Geometry check sheet. Reference: the model listing, model coordinates, mm. Face numbers are marked on the shaded views. Give positions to 0.01 mm unless a question says otherwise; leave off trailing zeros. Order: outer loops, then holes, each group sorted by start corner. A loop starts at its lowest first (then second) coordinate and runs counter-clockwise, first axis right, second up. Notation, with made-up numbers: M -17,-4.75 L -6,-4.75 A17 ccw -6,16.25 Z; hole C -21.5,29.5 d1. An arc over 180 degrees is marked long. Answer as CSV lines item,"result". Start each with the question number.
Q1. Section check A-A, the plane x = 0. Record the boundary of the cut face in (y, z).
Q2. Mould release check, pull along X, two halves, no side actions. Record for the marked faces 1 and 2: +X half, -X half, draft (parallel to the pull), parting line (faces both ways), or undercut.
Q3. Section check D-D, the plane x = -21. Record the boundary of the cut face in (y, z).
Q4. Go/stop test with flat-tipped pins: pin 1 (1.6 mm diameter, centred on x = 25.98, y = -15, fed in from +Z); pin 2 (1.5 mm diameter, centred on y = -19.5, z = 0.5, fed in from -X); pin 3 (2.5 mm diameter, centred on x = 0, y = 30, fed in from -Z). Record where each tip stops, or that it passes through.
Q5. Section check C-C, the plane y = -15. Count the separate pieces of the cut face and the enclosed holes in it, then the cut area to 3 significant figures.
Q6. Section check B-B, the plane y = 30. Record the boundary of the cut face in (x, z), then the cut area to 3 significant figures.
Q7. Thickness scan on line 1 (Y direction, x = 0, z = 3); line 2 (Y direction, x = 0, z = 0.3); line 3 (Z direction, x = 34, y = -8). Record the ranges inside material, lowest first.
```python
from build123d import *

# Parameters (mm, degrees)
SKETCH_1_R          = 40
EXTRUDE_1_DEPTH     = 4
SHELL_1_T           = -2
SKETCH_2_R          = 2
SKETCH_2_R_2        = 1
EXTRUDE_2_DEPTH     = 2
SKETCH_3_R          = 1
CUT_EXTRUDE_1_DEPTH = 20
SKETCH_4_R          = 1.6
CUT_EXTRUDE_2_DEPTH = 1.2


with BuildPart() as part:
    # 草图1 → 凸台-拉伸1 (new body)
    with BuildSketch(Plane.XY):
        Circle(SKETCH_1_R)
    extrude(amount=EXTRUDE_1_DEPTH)

    # 抽壳1
    shell_1_openings = [part.faces().sort_by_distance(p)[0] for p in [
        (0, 0, 4),
    ]]
    offset(amount=SHELL_1_T, openings=shell_1_openings, kind=Kind.INTERSECTION)

    # 草图2 → 凸台-拉伸2 (add)
    with BuildSketch(Plane.XY.offset(2)):
        with Locations((0, 30)):
            Circle(SKETCH_2_R)
        with Locations((0, 30)):
            Circle(SKETCH_2_R_2, mode=Mode.SUBTRACT)
        with Locations((25.980762114, -15)):
            Circle(SKETCH_2_R)
        with Locations((25.980762114, -15)):
            Circle(SKETCH_2_R_2, mode=Mode.SUBTRACT)
        with Locations((-25.980762114, -15)):
            Circle(SKETCH_2_R)
        with Locations((-25.980762114, -15)):
            Circle(SKETCH_2_R_2, mode=Mode.SUBTRACT)
    extrude(amount=EXTRUDE_2_DEPTH)

    # 草图3 → 切除-拉伸1 (cut)
    with BuildSketch(Plane.XY.offset(4)):
        with Locations((25.980762114, -15)):
            Circle(SKETCH_3_R)
        with Locations((-25.980762114, -15)):
            Circle(SKETCH_3_R)
        with Locations((0, 30)):
            Circle(SKETCH_3_R)
    extrude(amount=-CUT_EXTRUDE_1_DEPTH, mode=Mode.SUBTRACT)

    # 草图4 → 切除-拉伸2 (cut)
    with BuildSketch(Plane(origin=(0, 0, 0), x_dir=(-1, 0, 0), z_dir=(0, 0, -1))):
        with Locations((-25.980762114, -15)):
            Circle(SKETCH_4_R)
        with Locations((0, 30)):
            Circle(SKETCH_4_R)
        with Locations((25.980762114, -15)):
            Circle(SKETCH_4_R)
    extrude(amount=-CUT_EXTRUDE_2_DEPTH, mode=Mode.SUBTRACT)


solid = part.part
```
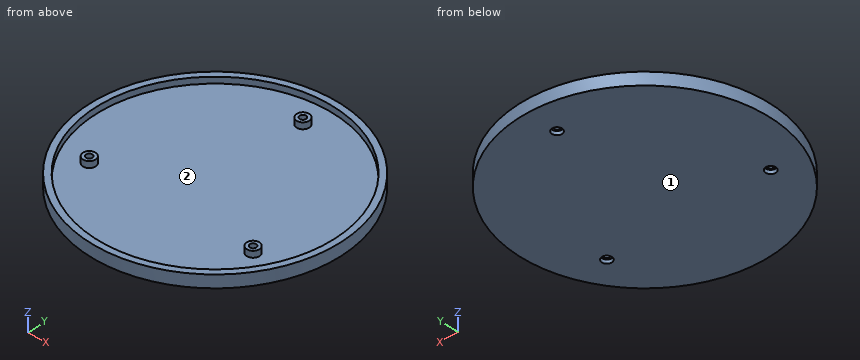
Answer block:
1,outline,"M -40,0 L 28.4,0 L 28.4,1.2 L 29,1.2 L 29,4 L 28,4 L 28,2 L -38,2 L -38,4 L -40,4 Z; M 31,1.2 L 31.6,1.2 L 31.6,0 L 40,0 L 40,4 L 38,4 L 38,2 L 32,2 L 32,4 L 31,4 Z"
2,face 1,"draft"
2,face 2,"undercut"
3,outline,"M -34.04,0 L 34.04,0 L 34.04,4 L 31.67,4 L 31.67,2 L -31.67,2 L -31.67,4 L -34.04,4 Z"
4,pin 1,"passes through"
4,pin 2,"stops at x = -35.33"
4,pin 3,"stops at z = 1.2"
5,separate pieces,"3"
5,enclosed holes,"0"
5,area,"154 mm2"
6,outline,"M -26.46,0 L -1.6,0 L -1.6,1.2 L -1,1.2 L -1,4 L -2,4 L -2,2 L -23.32,2 L -23.32,4 L -26.46,4 Z; M 1,1.2 L 1.6,1.2 L 1.6,0 L 26.46,0 L 26.46,4 L 23.32,4 L 23.32,2 L 2,2 L 2,4 L 1,4 Z"
6,area,"117 mm2"
7,line 1,"y = -40 to -38, 28 to 29, 31 to 32, 38 to 40"
7,line 2,"y = -40 to 28.4, 31.6 to 40"
7,line 3,"z = 0 to 2"
